from build123d import *

# Parameters (mm, degrees)
F0_R     = 6
F1_DEPTH = 25
F2_R     = 6
F3_W     = 7.4530789975
F3_H     = 13.9023570546
F4_DEPTH = 12.5
F5_W     = 5.4
F5_H     = 5.4
F6_DEPTH = 25
F7_W     = 5.4
F7_H     = 5.4
F7_W_2   = 4.6
F7_H_2   = 4.6
F8_DEPTH = 1
F9_R     = 0.19999


# Not quite as in the source:
# - a fillet or chamfer is up to 0.001 mm smaller than in the source, because OpenCascade refuses the exact size


with BuildPart() as f1:
    # F0 (on Top) → F1 (new body)
    with BuildSketch(Plane.XY):
        Circle(F0_R)
    extrude(amount=F1_DEPTH)

    # F2
    f2_edges = [f1.edges().sort_by_distance(p)[0] for p in [
        (-6, 0, 25),
    ]]
    fillet(f2_edges, radius=F2_R)

    # F3 (on Front) → F4 (cut, symmetric)
    with BuildSketch(Plane.XZ):
        with Locations((3.7265394987, 19.9511785273)):
            Rectangle(F3_W, F3_H)
    extrude(amount=F4_DEPTH, both=True, mode=Mode.SUBTRACT)

    # F5 (on face) → F6 (cut)
    with BuildSketch(Plane.YZ):
        with Locations((0, 18.7)):
            Rectangle(F5_W, F5_H)
    extrude(amount=-F6_DEPTH, mode=Mode.SUBTRACT)

    # F7 (on face) → F8 (join)
    with BuildSketch(Plane.YZ):
        with Locations((0, 18.7)):
            Rectangle(F7_W, F7_H)
        with Locations((0, 18.7)):
            Rectangle(F7_W_2, F7_H_2, mode=Mode.SUBTRACT)
    extrude(amount=-F8_DEPTH)

    # F9 (radius 0.2 in the source; OpenCascade refuses exactly that, so slightly less here)
    f9_edges = [f1.edges().sort_by_distance(p)[0] for p in [
        (-1, 0, 16.4),
        (-1, 2.3, 18.7),
        (-1, 0, 21),
        (-1, -2.3, 18.7),
        (-1, 0, 21.4),
        (-1, -2.7, 18.7),
        (-1, 2.7, 18.7),
        (-1, 0, 16),
    ]]
    fillet(f9_edges, radius=F9_R)

    # F10: F1 across plane


with BuildPart() as f1_1:
    add(f1.part)
    add(f1.part.mirror(Plane.XY))


solid = f1_1.part
Could you check a few things on this model? Use its own coordinates, in mm. A direction names the side the tool comes from. Round coordinates to 2 decimals unless told otherwise and drop trailing zeros. Write each loop counter-clockwise with the first axis right and the second up, starting at its lowest first coordinate (ties: lowest second). Pieces come first, ordered by that corner, then holes. Notation, with made-up numbers: (35.25, -14.5) -> (77.25, -14.5) arc R22 ccw to (77.25, 2.5) -> close; hole circle Ø7 at (-22, -35). An arc over 180 degrees is marked (long way). Use a Markdown table: item, result.
1. Which directions (+Z, -Z, +X, -X, +Y, -Y) give clear straight access to the entire face, cutting with the end or side of a thin tool? Please do faces 3 (the face through (-0.4, 2.3, 18.7)), 4 (the face through (2, 0, -13)), 5 (the face through (-3, -2.7, -19)).
Answer key:
| item | result |
|---|---|
| face 3 | +X, -X |
| face 4 | -Z, +X, +Y, -Y |
| face 5 | -X |
2. If we section it at D-D (x = 2.5): List the corners of the cut face in (y, z) for me.
Answer key:
| item | result |
|---|---|
| outline | (-5.45, -13) -> (5.45, -13) -> (5.45, 13) -> (-5.45, 13) -> close |
3. We'd pull the mould along Y, two halves only. Please class faces 1 (the face through (0, 3, -19)), 2 (the face through (-4, 0, -16)): +Y half, -Y half, draft (parallel to the pull), parting line (faces both ways), or undercut.
Answer key:
| item | result |
|---|---|
| face 1 | draft |
| face 2 | undercut |
4. If we section it at C-C (y = -4.75): List the corners of the cut face in (x, z) for me.
Answer key:
| item | result |
|---|---|
| outline | (-3.67, -19) arc R3.67 ccw to (0, -22.67) -> (0, -13) -> (3.67, -13) -> (3.67, 13) -> (0, 13) -> (0, 22.67) arc R3.67 ccw to (-3.67, 19) -> close |
5. For pin 1 Ø4.5 at (x, y) = (-4, 0) entering from +Z; pin 2 Ø0.6 at (x, y) = (-0.5, 0.5) entering from -Z; pin 3 Ø0.6 at (x, z) = (-0.5, -17.5) entering from +Y, each with a flat end and sliding along its axis, tell me the tip position at first contact or that it passes through.
Answer key:
| item | result |
|---|---|
| pin 1 | stops at z = 24.74 |
| pin 2 | stops at z = -24.99 |
| pin 3 | stops at y = 6 |
6. If we section it at B-B (x = -2): List the corners of the cut face in (y, z) for me, then the cut area to 3 significant figures.
Answer key:
| item | result |
|---|---|
| outline | (-5.66, -19) arc R5.66 ccw to (5.66, -19) -> (5.66, 19) arc R5.66 ccw to (-5.66, 19) -> close; hole (-2.7, -21.4) -> (2.7, -21.4) -> (2.7, -16) -> (-2.7, -16) -> close; hole (-2.7, 16) -> (2.7, 16) -> (2.7, 21.4) -> (-2.7, 21.4) -> close |
| area | 472 mm^2 |
7. Please list where these lines run through material, in increasing order: probe 1 along Z at (x, y) = (-3, -0.25); probe 2 along Z at (x, y) = (2, -1); probe 3 along Z at (x, y) = (-1.75, -0.75).
Answer key:
| item | result |
|---|---|
| probe 1 | z = -24.19 to -21.4, -16 to 16, 21.4 to 24.19 |
| probe 2 | z = -13 to 13 |
| probe 3 | z = -24.69 to -21.4, -16 to 16, 21.4 to 24.69 |
8. If we section it at A-A (y = 0): State how many separate pieces and enclosed holes the cut face has, then the cut area to 3 significant figures.
Answer key:
| item | result |
|---|---|
| separate pieces | 3 |
| enclosed holes | 0 |
| area | 378 mm^2 |
